Source: CAD feature listing. Evaluate the final solid. Frame: model axes, mm. Face numbers are marked on the shaded views. Give positions to 0.01 mm unless a question says otherwise; leave off trailing zeros. Loops run counter-clockwise (first coordinate to the right, second up) from the corner with the lowest first, then second, coordinate; pieces in that order, holes last. Notation, with made-up numbers: (-16, -31.5) - (24, -31.5) arc R19 ccw to (24, 1.5) - close; hole circle Ø8 at (-33, -39). An arc over 180 degrees is marked (long way). Put each result on its own line as item: value.
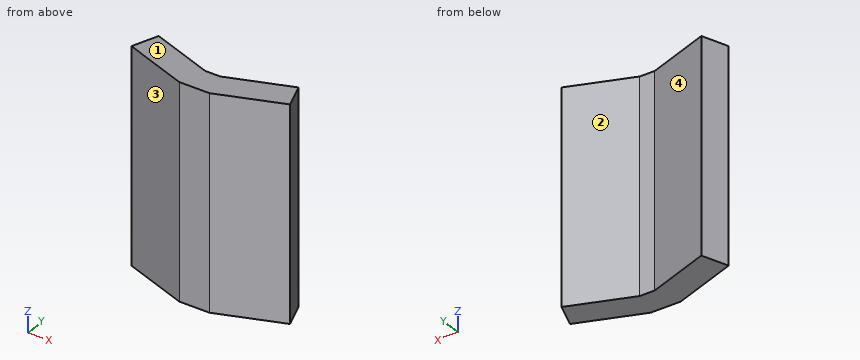
```python
from build123d import *

# Parameters (mm, degrees)
BOSS_EXTRUDE2_DEPTH      = 77.5
BOSS_EXTRUDE2_DEPTH_BACK = 77.5


with BuildPart() as part:
    # Sketch7 → Boss-Extrude2 (new, two sides: drawn at the far end of the back side and taken through both)
    with BuildSketch(Plane.XY.offset(-BOSS_EXTRUDE2_DEPTH_BACK)):
        Polygon((-11, 0), (11, 0), (57.984631039, 17.101007166), (51.144228173, 35.894859582), (5.462206168, 19.267963331), (-5.462206168, 19.267963331), (-51.144228173, 35.894859582), (-57.984631039, 17.101007166), align=None)
    extrude(amount=BOSS_EXTRUDE2_DEPTH + BOSS_EXTRUDE2_DEPTH_BACK)


solid = part.part
```
1) Section query B-B, the plane z = 36.5. Output: boundary loops of the cut face in (x, y).
Check result:
outline: (-57.98, 17.1) - (-11, 0) - (11, 0) - (57.98, 17.1) - (51.14, 35.89) - (5.46, 19.27) - (-5.46, 19.27) - (-51.14, 35.89) - close
2) Pin query (flat end, axial travel): P1, Ø12, axis at y = 22, z = 14, coming from the +X side; P2, Ø8, axis at y = 30.5, z = -52.5, coming from the -X side; P3, Ø3.5, axis at x = 0, z = 32.5, coming from the +Y side; P4, Ø10, axis at x = 26, z = 23.5, coming from the -Y side. Return the tip coordinate at first contact, or that it passes through.
Check result:
P1: x = 57.98
P2: x = -54.56
P3: y = 19.27
P4: y = 3.64
3) Section query A-A, the plane y = 32.5. Output: boundary loops of the cut face in (x, z), plus the area to 3 significant figures.
Check result:
outline: (-52.38, -77.5) - (-41.82, -77.5) - (-41.82, 77.5) - (-52.38, 77.5) - close; (41.82, -77.5) - (52.38, -77.5) - (52.38, 77.5) - (41.82, 77.5) - close
area: 3,270 mm²
4) Mould query, pull axis X, two halves, no side actions, for the marked faces 1, 2, 3 and 4. Classes: pulls with the +X half, pulls with the -X half, needs draft (parallel to the pull), parting line crosses it, or undercut.
Check result:
face 1: needs draft
face 2: undercut
face 3: pulls with the -X half
face 4: undercut
5) Section query D-D, the plane y = 23. Output: boundary loops of the cut face in (x, z).
Check result:
outline: (-55.84, -77.5) - (-15.72, -77.5) - (-15.72, 77.5) - (-55.84, 77.5) - close; (15.72, -77.5) - (55.84, -77.5) - (55.84, 77.5) - (15.72, 77.5) - close
6) Material intervals for line 1 along Y through (x, z) = (-5, 48.5); line 2 along Y through (x, z) = (-20, -6), sorted ascending. Write a range as [from, to].
Check result:
line 1: [0, 19.27]
line 2: [3.28, 24.56]
7) Section query C-C, the plane x = 2.5. Output: boundary loops of the cut face in (y, z), plus the area to 3 significant figures.
Check result:
outline: (0, -77.5) - (19.27, -77.5) - (19.27, 77.5) - (0, 77.5) - close
area: 2,990 mm²
